from build123d import *

# Parameters (mm, degrees)
SKIZZE1_R                                           = 50
AUFSATZ_LINEAR_AUSTRAGEN1_DEPTH                     = 200
STIRNSENKUNG_F_R_M8_SENKSCHRAUBE_KOPF_B_D           = 9
STIRNSENKUNG_F_R_M8_SENKSCHRAUBE_KOPF_B_CBORE_D     = 22
STIRNSENKUNG_F_R_M8_SENKSCHRAUBE_KOPF_B_CBORE_DEPTH = 8
STIRNSENKUNG_F_R_M8_SENKSCHRAUBE_KO_2_D             = 9
STIRNSENKUNG_F_R_M8_SENKSCHRAUBE_KO_2_CBORE_D       = 15
STIRNSENKUNG_F_R_M8_SENKSCHRAUBE_KO_2_CBORE_DEPTH   = 8


with BuildPart() as part:
    # Skizze1 → Aufsatz-Linear austragen1 (new body)
    with BuildSketch(Plane.XY):
        Circle(SKIZZE1_R)
    extrude(amount=AUFSATZ_LINEAR_AUSTRAGEN1_DEPTH)

    # Stirnsenkung f_r M8 Senkschraube _Kopf B (through all)
    with Locations(Plane(origin=(0, 50, 0), x_dir=(1, 0, 0), z_dir=(0, 1, 0))):
        with Locations((0, -25), (0, -175)):
            CounterBoreHole(STIRNSENKUNG_F_R_M8_SENKSCHRAUBE_KOPF_B_D / 2, STIRNSENKUNG_F_R_M8_SENKSCHRAUBE_KOPF_B_CBORE_D / 2, STIRNSENKUNG_F_R_M8_SENKSCHRAUBE_KOPF_B_CBORE_DEPTH)

    # Stirnsenkung f_r M8 Senkschraube _Ko 2 (through all)
    with Locations(Plane(origin=(0, -50, 0), x_dir=(-1, 0, 0), z_dir=(0, -1, 0))):
        with Locations((0, -175), (0, -25)):
            CounterBoreHole(STIRNSENKUNG_F_R_M8_SENKSCHRAUBE_KO_2_D / 2, STIRNSENKUNG_F_R_M8_SENKSCHRAUBE_KO_2_CBORE_D / 2, STIRNSENKUNG_F_R_M8_SENKSCHRAUBE_KO_2_CBORE_DEPTH)


solid = part.part
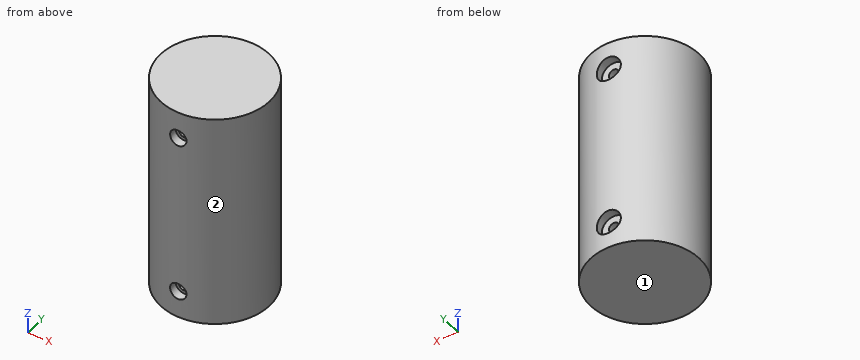
Input: part model. Units: mm. Frame: model coordinates. Face numbers are marked on the shaded views. Round coordinates to 2 decimals unless told otherwise and drop trailing zeros. Loops run counter-clockwise (first coordinate to the right, second up) from the corner with the lowest first, then second, coordinate; pieces in that order, holes last. Notation, with made-up numbers: (50, 29.25) -> (73, 29.25) arc R24 ccw to (73, 47.25) -> close; hole circle Ø5 at (62.25, 33.5). An arc over 180 degrees is marked (long way). Answer as a JSON object with one key per item and string values. Group by question number.
1) Section query C-C on y = -27.5. Output: boundary loops of the cut face in (x, z), plus the area to 3 significant figures.
2) Pin query (flat end, axial travel): pin 1 (12 mm diameter, centred on x = 10, z = 24.5, fed in from +Y); pin 2 (17 mm diameter, centred on x = 0, z = 25, fed in from -Y); pin 3 (5 mm diameter, centred on x = 28, z = 27.5, fed in from -Y); pin 4 (2 mm diameter, centred on y = 34, z = 152.5, fed in from -X). Return the tip coordinate at first contact, or that it passes through.
3) Draft query along Y for the marked faces 1 and 2. Return one class per face: +Y half, -Y half, draft (parallel to the pull), parting line (faces both ways), or undercut.
4) Section query D-D on z = 54. Output: boundary loops of the cut face in (x, y).
5) Ray query, L1, parallel to Z at x = 0, y = -46; L2, parallel to Z at x = 0, y = 46.25; L3, parallel to X at y = -44.25, z = 175. Return the intervals inside material, ascending.
6) Section query A-A on x = 0. Output: boundary loops of the cut face in (y, z), plus the area to 3 significant figures.
7) Section query B-B on z = 175. Output: boundary loops of the cut face in (x, y) (3 decimals), plus the area to 3 significant figures.
Reply:
{
 "1": {"outline": "(-41.76, 0) -> (41.76, 0) -> (41.76, 200) -> (-41.76, 200) -> close; hole circle Ø9 at (0, 25); hole circle Ø9 at (0, 175)", "area": "16,600 mm2"},
 "2": {"pin 1": "stops at y = 49.19", "pin 2": "stops at y = -50", "pin 3": "stops at y = -43.01", "pin 4": "stops at x = -37.56"},
 "3": {"face 1": "draft", "face 2": "parting line"},
 "4": {"outline": "circle Ø100 at (0, 0)"},
 "5": {"L1": "z = 0 to 17.5, 32.5 to 167.5, 182.5 to 200", "L2": "z = 0 to 14, 36 to 164, 186 to 200", "L3": "x = -23.28 to -7.5, 7.5 to 23.28"},
 "6": {"outline": "(-50, 0) -> (50, 0) -> (50, 14) -> (42, 14) -> (42, 20.5) -> (-42, 20.5) -> (-42, 17.5) -> (-50, 17.5) -> close; (-50, 32.5) -> (-42, 32.5) -> (-42, 29.5) -> (42, 29.5) -> (42, 36) -> (50, 36) -> (50, 164) -> (42, 164) -> (42, 170.5) -> (-42, 170.5) -> (-42, 167.5) -> (-50, 167.5) -> close; (-50, 182.5) -> (-42, 182.5) -> (-42, 179.5) -> (42, 179.5) -> (42, 186) -> (50, 186) -> (50, 200) -> (-50, 200) -> close", "area": "17,900 mm2"},
 "7": {"outline": "(-11, 42) -> (-11, 48.775) arc R50 ccw to (-7.5, -49.434) -> (-7.5, -42) -> (-4.5, -42) -> (-4.5, 42) -> close; (4.5, -42) -> (7.5, -42) -> (7.5, -49.434) arc R50 ccw to (11, 48.775) -> (11, 42) -> (4.5, 42) -> close", "area": "6,810 mm2"}
}
